Part model, mm, in its own coordinate system. Round coordinates to 2 decimals unless told otherwise and drop trailing zeros. Write each loop counter-clockwise with the first axis right and the second up, starting at its lowest first coordinate (ties: lowest second). Pieces come first, ordered by that corner, then holes. Notation, with made-up numbers: M -22,-36 L 14,-36 A14 cw 14,-29 Z; hole C -3,11.25 d3. An arc over 180 degrees is marked long. One line per question, with ' | ' between items. Start each with the question number.
1) Wall check: probe 1 along X at (y, z) = (1.7, 3.5); probe 2 along Z at (x, y) = (46, 1.2); probe 3 along Y at (x, z) = (19, 3.2). Give the ranges that are in metal, low to high. Write a range as [from, to].
2) Saw through at A-A (x = 7.5). List the corners of the cut face in (y, z).
3) Drop flat-ended pins along their axis: pin 1 Ø1 at (y, z) = (-0.5, 1) entering from +X; pin 2 Ø0.6 at (y, z) = (-1.5, 2.5) entering from +X; pin 3 Ø0.6 at (y, z) = (0.5, 1) entering from -X. Give the stop position or say it passes through.
```python
from build123d import *

# Parameters (mm, degrees)
F0_W     = 146
F0_H     = 4
F1_DEPTH = 4
F3_DEPTH = 12
F6_DEPTH = 12
F8_R     = 1


# Not quite as in the source:
# - a fillet or chamfer that OpenCascade refuses, or shapes differently, is made with other operations: its cross-section is extruded or revolved along the edge and cut away or added


with BuildPart() as f1:
    # F0 (on Top) → F1 (new body)
    with BuildSketch(Plane.XY):
        Rectangle(F0_W, F0_H)
    extrude(amount=F1_DEPTH)

    # F2 (on face) → F3 (join)
    with BuildSketch(Plane(origin=(-73, 0, 0), x_dir=(0, -1, 0), z_dir=(-1, 0, 0))):
        with BuildLine():
            ThreePointArc((0, 0), (1.4142135624, 0.5857864376), (2, 2))
            ThreePointArc((2, 2), (1.4142135624, 3.4142135624), (0, 4))
            ThreePointArc((0, 4), (-1.4142135624, 3.4142135624), (-2, 2))
            ThreePointArc((-2, 2), (-1.4142135624, 0.5857864376), (0, 0))
        make_face()
    extrude(amount=F3_DEPTH)

    # F4: fillet of radius 2 on 1 edges, made by hand

    # F4_s1 → F4_t2 (revolve, cut)
    with BuildSketch(Plane.XZ):
        with BuildLine():
            ThreePointArc((-83, 0), (-84.4142135624, 0.5857864376), (-85, 2))
            Line((-85, 2), (-85, 0))
            Line((-85, 0), (-83, 0))
        make_face()
    revolve(axis=Axis((-85, 0, 2), (1, 0, 0)), mode=Mode.SUBTRACT)

    # F5 (on face) → F6 (join)
    with BuildSketch(Plane.YZ.offset(73)):
        with BuildLine():
            ThreePointArc((0, 0), (1.4142135624, 0.5857864376), (2, 2))
            ThreePointArc((2, 2), (1.4142135624, 3.4142135624), (0, 4))
            ThreePointArc((0, 4), (-1.4142135624, 3.4142135624), (-2, 2))
            ThreePointArc((-2, 2), (-1.4142135624, 0.5857864376), (0, 0))
        make_face()
    extrude(amount=F6_DEPTH)

    # F7: fillet of radius 2 on 1 edges, made by hand

    # F7_s1 → F7_t2 (revolve, cut)
    with BuildSketch(Plane.XZ):
        with BuildLine():
            ThreePointArc((83, 0), (84.4142135624, 0.5857864376), (85, 2))
            Line((85, 2), (85, 0))
            Line((85, 0), (83, 0))
        make_face()
    revolve(axis=Axis((85, 0, 2), (-1, 0, 0)), mode=Mode.SUBTRACT)

    # F8
    f8_edges = [f1.edges().sort_by_distance(p)[0] for p in [
        (0, -2, 4),
        (0, -2, 0),
        (0, 2, 0),
        (0, 2, 4),
    ]]
    fillet(f8_edges, radius=F8_R)


solid = f1.part
```
Answer key:
1) probe 1: x = [-73, 73] | probe 2: z = [0.02, 3.98] | probe 3: y = [-1.98, 1.98]
2) outline: M -2,1 A1 ccw -1,0 L 1,0 A1 ccw 2,1 L 2,3 A1 ccw 1,4 L -1,4 A1 ccw -2,3 Z
3) pin 1: stops at x = 84.9 | pin 2: stops at x = 84.54 | pin 3: stops at x = -84.83
